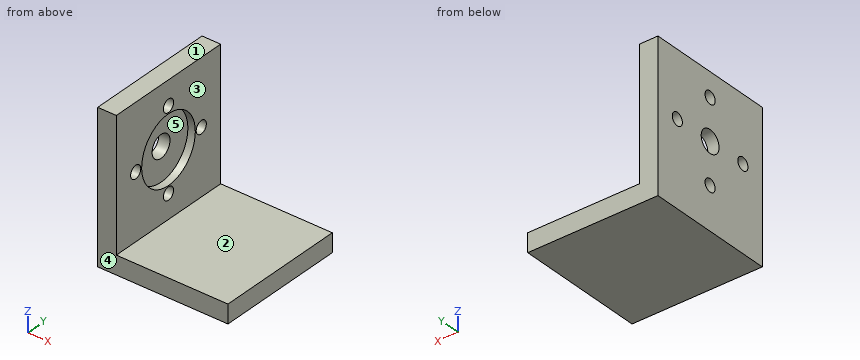
```python
from build123d import *

# Parameters (mm, degrees)
SKETCH3_W           = 35
SKETCH3_H           = 35
BOSS_EXTRUDE1_DEPTH = 5
SKETCH4_R           = 9
CUT_EXTRUDE1_DEPTH  = 2
SKETCH5_R           = 3
CUT_EXTRUDE2_DEPTH  = 25.929901725
SKETCH6_R           = 1.7
CUT_EXTRUDE3_DEPTH  = 26.248762346
SKETCH8_W           = 35
SKETCH8_H           = 35
BOSS_EXTRUDE2_DEPTH = 5


with BuildPart() as part:
    # Sketch3 → Boss-Extrude1 (new body)
    with BuildSketch(Plane.YZ):
        Rectangle(SKETCH3_W, SKETCH3_H)
    extrude(amount=BOSS_EXTRUDE1_DEPTH)

    # Sketch4 → Cut-Extrude1 (cut)
    with BuildSketch(Plane.YZ.offset(5)):
        with Locations(Location((0, 0, 0), (0, 0, 270))):
            Circle(SKETCH4_R)
    extrude(amount=-CUT_EXTRUDE1_DEPTH, mode=Mode.SUBTRACT)

    # Sketch5 → Cut-Extrude2 (cut, through all)
    with BuildSketch(Plane.YZ.offset(3)):
        with Locations(Location((0, 0, 0), (0, 0, 270))):
            Circle(SKETCH5_R)
    extrude(amount=-CUT_EXTRUDE2_DEPTH, mode=Mode.SUBTRACT)

    # Sketch6 → Cut-Extrude3 (cut, through all)
    with BuildSketch(Plane.YZ.offset(5)):
        with Locations(Location((0, 11, 0), (0, 0, 270))):
            Circle(SKETCH6_R)
        with Locations(Location((-11, 0, 0), (0, 0, 270))):
            Circle(SKETCH6_R)
        with Locations(Location((0, -11, 0), (0, 0, 270))):
            Circle(SKETCH6_R)
        with Locations(Location((11, 0, 0), (0, 0, 270))):
            Circle(SKETCH6_R)
    extrude(amount=-CUT_EXTRUDE3_DEPTH, mode=Mode.SUBTRACT)

    # Sketch8 → Boss-Extrude2 (add)
    with BuildSketch(Plane(origin=(0, 0, -17.5), x_dir=(1, 0, 0), z_dir=(0, 0, -1))):
        with Locations((17.5, 0)):
            Rectangle(SKETCH8_W, SKETCH8_H)
    extrude(amount=BOSS_EXTRUDE2_DEPTH)


solid = part.part
```
Verification items for the finished model (mm, model axes). Face numbers are marked on the shaded views. A direction names the side the tool comes from. Round coordinates to 2 decimals unless told otherwise and drop trailing zeros. Write each loop counter-clockwise with the first axis right and the second up, starting at its lowest first coordinate (ties: lowest second). Pieces come first, ordered by that corner, then holes. Notation, with made-up numbers: (42, 21.5) -> (59, 21.5) arc R20 ccw to (59, 31.5) -> close; hole circle Ø2 at (3, -36.5). An arc over 180 degrees is marked (long way). Write each question's results on one line, items separated by ' | '. Start each with the question number.
1. Depth check by flat-ended pin: P1, Ø4.5, axis at y = -11, z = 0, coming from the +X side; P2, Ø5.5, axis at y = 2, z = 4, coming from the +X side; P3, Ø4, axis at x = 23.5, y = -10.5, coming from the +Z side. Enter the tip coordinate at first touch or a pass-through.
2. Material ranges on probe 1 along Y at (x, z) = (0.85, 0); probe 2 along Y at (x, z) = (4.25, 0); probe 3 along Y at (x, z) = (1.1, -11), recorded low to high. Write a range as from..to.
3. Cross-section at A-A (z = 0). Enter the section's corners in (x, y).
4. Set-up check for the marked faces 1 and 2: record each of +Z, -Z, +X, -X, +Y, -Y from which the full face is reachable in a straight line by a thin tool's end or side.
5. Draft check along Y on the marked faces 3, 4 and 5. Enter one of: +Y half, -Y half, draft (parallel to the pull), parting line (faces both ways), or undercut.
6. Cross-section at D-D (y = 0). Enter the section's corners in (x, z).
7. Cross-section at C-C (z = -11). Enter the section's corners in (x, y).
8. Cross-section at B-B (y = -11). Enter the section's corners in (x, z), then the cut area to 3 significant figures.
Solutions:
1) P1: stops at x = 5 | P2: stops at x = 3 | P3: stops at z = -17.5
2) probe 1: y = -17.5..-12.7, -9.3..-3, 3..9.3, 12.7..17.5 | probe 2: y = -17.5..-12.7, -9.3..-9, 9..9.3, 12.7..17.5 | probe 3: y = -17.5..-1.7, 1.7..17.5
3) outline: (0, -17.5) -> (5, -17.5) -> (5, -12.7) -> (0, -12.7) -> close; (0, -9.3) -> (5, -9.3) -> (5, -9) -> (3, -9) -> (3, -3) -> (0, -3) -> close; (0, 3) -> (3, 3) -> (3, 9) -> (5, 9) -> (5, 9.3) -> (0, 9.3) -> close; (0, 12.7) -> (5, 12.7) -> (5, 17.5) -> (0, 17.5) -> close
4) face 1: +Z, +X, -X, +Y, -Y | face 2: +Z, +X, +Y, -Y
5) face 3: draft | face 4: -Y half | face 5: undercut
6) outline: (0, -22.5) -> (35, -22.5) -> (35, -17.5) -> (5, -17.5) -> (5, -12.7) -> (0, -12.7) -> close; (0, -9.3) -> (5, -9.3) -> (5, -9) -> (3, -9) -> (3, -3) -> (0, -3) -> close; (0, 3) -> (3, 3) -> (3, 9) -> (5, 9) -> (5, 9.3) -> (0, 9.3) -> close; (0, 12.7) -> (5, 12.7) -> (5, 17.5) -> (0, 17.5) -> close
7) outline: (0, -17.5) -> (5, -17.5) -> (5, -1.7) -> (0, -1.7) -> close; (0, 1.7) -> (5, 1.7) -> (5, 17.5) -> (0, 17.5) -> close
8) outline: (0, -22.5) -> (35, -22.5) -> (35, -17.5) -> (5, -17.5) -> (5, -1.7) -> (0, -1.7) -> close; (0, 1.7) -> (5, 1.7) -> (5, 17.5) -> (0, 17.5) -> close | area: 333 mm2
